```python
from build123d import *

# Parameters (mm, degrees)
SKETCH_1_W          = 158
SKETCH_1_H          = 48
EXTRUDE_1_DEPTH     = 2
SKETCH_2_W          = 128
SKETCH_2_H          = 28
CUT_EXTRUDE_1_DEPTH = 2
SKETCH_4_R          = 1.7
CUT_EXTRUDE_2_DEPTH = 2
SKETCH_5_R          = 1.6
CUT_EXTRUDE_3_DEPTH = 2
FILLET_4_R          = 3
FILLET_5_R          = 4
FILLET_6_R          = 20


with BuildPart() as part:
    # 草图1 → 凸台-拉伸1 (new body)
    with BuildSketch(Plane(origin=(0, 0, 0), x_dir=(1, 0, 0), z_dir=(0, 1, 0))):
        Rectangle(SKETCH_1_W, SKETCH_1_H)
    extrude(amount=EXTRUDE_1_DEPTH)

    # 草图2 → 切除-拉伸1 (cut)
    with BuildSketch(Plane(origin=(0, 2, 0), x_dir=(1, 0, 0), z_dir=(0, 1, 0))):
        with Locations((0, -10)):
            Rectangle(SKETCH_2_W, SKETCH_2_H)
    extrude(amount=-CUT_EXTRUDE_1_DEPTH, mode=Mode.SUBTRACT)

    # 草图4 → 切除-拉伸2 (cut)
    with BuildSketch(Plane(origin=(0, 2, 0), x_dir=(1, 0, 0), z_dir=(0, 1, 0))):
        with Locations(Location((-74, 19.85, 0), (0, 0, 270))):
            Circle(SKETCH_4_R)
        with Locations(Location((-74, -9.65, 0), (0, 0, 270))):
            Circle(SKETCH_4_R)
        with Locations(Location((-74, -20.15, 0), (0, 0, 270))):
            Circle(SKETCH_4_R)
        with Locations(Location((74, -20.15, 0), (0, 0, 90))):
            Circle(SKETCH_4_R)
        with Locations(Location((74, -9.65, 0), (0, 0, 90))):
            Circle(SKETCH_4_R)
        with Locations(Location((74, 19.85, 0), (0, 0, 90))):
            Circle(SKETCH_4_R)
    extrude(amount=-CUT_EXTRUDE_2_DEPTH, mode=Mode.SUBTRACT)

    # 草图5 → 切除-拉伸3 (cut)
    with BuildSketch(Plane(origin=(0, 2, 0), x_dir=(1, 0, 0), z_dir=(0, 1, 0))):
        with Locations(Location((0, 14, 0), (0, 0, 270))):
            Circle(SKETCH_5_R)
        with Locations(Location((-45, 14, 0), (0, 0, 270))):
            Circle(SKETCH_5_R)
        with Locations(Location((45, 14, 0), (0, 0, 270))):
            Circle(SKETCH_5_R)
    extrude(amount=-CUT_EXTRUDE_3_DEPTH, mode=Mode.SUBTRACT)

    # 圆角4
    fillet_4_edges = [part.edges().sort_by_distance(p)[0] for p in [
        (79, 1, 24),
        (-79, 1, 24),
        (-79, 1, -24),
        (79, 1, -24),
    ]]
    fillet(fillet_4_edges, radius=FILLET_4_R)

    # 圆角5
    fillet_5_edges = [part.edges().sort_by_distance(p)[0] for p in [
        (64, 1, 24),
        (-64, 1, 24),
    ]]
    fillet(fillet_5_edges, radius=FILLET_5_R)

    # 圆角6
    fillet_6_edges = [part.edges().sort_by_distance(p)[0] for p in [
        (64, 1, -4),
        (-64, 1, -4),
    ]]
    fillet(fillet_6_edges, radius=FILLET_6_R)


solid = part.part
```
Geometry: final body of the model. Coordinates: model frame, mm. A direction names the side the tool comes from. Round coordinates to 2 decimals unless told otherwise and drop trailing zeros. Order: outer loops, then holes, each group sorted by start corner. A loop starts at its lowest first (then second) coordinate and runs counter-clockwise, first axis right, second up. Notation, with made-up numbers: M 0,1 L 42,1 A17 cw 42,12 Z; hole C 10,88 d11. An arc over 180 degrees is marked long. One line per item, written item: value.
(1) Line query: probe 1 along Z at (x, y) = (-74, 1.2); probe 2 along X at (y, z) = (0.75, -14); probe 3 along X at (y, z) = (1.55, -19.85). Output: solid intervals per line, ascending. Write a range as [from, to].
Result sheet:
probe 1: [-24, -21.55], [-18.15, 7.95], [11.35, 18.45], [21.85, 24]
probe 2: [-79, -46.6], [-43.4, -1.6], [1.6, 43.4], [46.6, 79]
probe 3: [-79, -75.7], [-72.3, 72.3], [75.7, 79]
(2) Cut plane D-D (x = 74). Return the cut outline in (y, z), and give its area (3 significant figures).
Result sheet:
outline: M 0,-24 L 2,-24 L 2,-21.55 L 0,-21.55 Z; M 0,-18.15 L 2,-18.15 L 2,7.95 L 0,7.95 Z; M 0,11.35 L 2,11.35 L 2,18.45 L 0,18.45 Z; M 0,21.85 L 2,21.85 L 2,24 L 0,24 Z
area: 75.6 mm2
(3) Cut plane C-C (y = 0.3). Give the number of separate pieces and of enclosed holes in the cut face, and give its area (3 significant figures).
Result sheet:
separate pieces: 1
enclosed holes: 9
area: 4,080 mm2
(4) Cut plane A-A (x = 0). Return the cut outline in (y, z).
Result sheet:
outline: M 0,-24 L 2,-24 L 2,-15.6 L 0,-15.6 Z; M 0,-12.4 L 2,-12.4 L 2,-4 L 0,-4 Z
(5) Reachability of faces 5 (the cylindrical face through (73.93, 1.01, -18.15)), 6 (the cylindrical face through (65.141, 0.986, 22.797)) from +Z, -Z, +X, -X, +Y, -Y: full face, straight path, thin tool, end or side. Return the list, or none.
Result sheet:
face 5: +Y, -Y
face 6: +Z, +Y, -Y
(6) Cut plane B-B (z = 9.65). Return the cut outline in (x, y), and give its area (3 significant figures).
Result sheet:
outline: M -79,0 L -75.7,0 L -75.7,2 L -79,2 Z; M -72.3,0 L -62.97,0 L -62.97,2 L -72.3,2 Z; M 62.97,0 L 72.3,0 L 72.3,2 L 62.97,2 Z; M 75.7,0 L 79,0 L 79,2 L 75.7,2 Z
area: 50.5 mm2
(7) Pull-direction query (X, two-part tool) for faces 1 (the flat face through (-1, 0, -11)), 2 (the cylindrical face through (-75.03, 1.01, 8.3)), 3 (the cylindrical face through (73.93, 1.01, 21.85)), 4 (the cylindrical face through (-78.14, 1.01, -23.1)); classes: pulls with the +X half, pulls with the -X half, needs draft (parallel to the pull), parting line crosses it, or undercut.
Result sheet:
face 1: needs draft
face 2: undercut
face 3: undercut
face 4: pulls with the -X half
